from build123d import *

# Parameters (mm, degrees)
F1_DEPTH = 4
F2_R     = 3.5
F2_R_2   = 1.05
F3_DEPTH = 3


with BuildPart() as f1:
    # F0 (on Top) → F1 (new body)
    with BuildSketch(Plane.XY):
        with BuildLine():
            Line((2.511473671, -1.45), (2.511473671, 1.45))
            Line((2.511473671, 1.45), (0, 2.9))
            Line((0, 2.9), (0, 1.05))
            ThreePointArc((0, 1.05), (0.7424621202, 0.7424621202), (1.05, 0))
            ThreePointArc((1.05, 0), (0.7424621202, -0.7424621202), (0, -1.05))
            Line((0, -1.05), (0, -2.9))
            Line((0, -2.9), (2.511473671, -1.45))
        make_face()
        with BuildLine():
            Line((0, 1.05), (0, 2.9))
            Line((0, 2.9), (-2.511473671, 1.45))
            Line((-2.511473671, 1.45), (-2.511473671, -1.45))
            Line((-2.511473671, -1.45), (0, -2.9))
            Line((0, -2.9), (0, -1.05))
            ThreePointArc((0, -1.05), (-1.05, 0), (0, 1.05))
        make_face()
    extrude(amount=F1_DEPTH)

    # F2 (on face) → F3 (join)
    with BuildSketch(Plane(origin=(0, 0, 0), x_dir=(1, 0, 0), z_dir=(0, 0, -1))):
        Circle(F2_R)
        Polygon((0, 2.9), (2.511473671, 1.45), (2.511473671, -1.45), (0, -2.9), (-2.511473671, -1.45), (-2.511473671, 1.45), align=None, mode=Mode.SUBTRACT)
        Polygon((2.511473671, -1.45), (2.511473671, 1.45), (0, 2.9), (-2.511473671, 1.45), (-2.511473671, -1.45), (0, -2.9), align=None)
        Circle(F2_R_2, mode=Mode.SUBTRACT)
        Circle(F2_R_2)
    extrude(amount=F3_DEPTH)


solid = f1.part
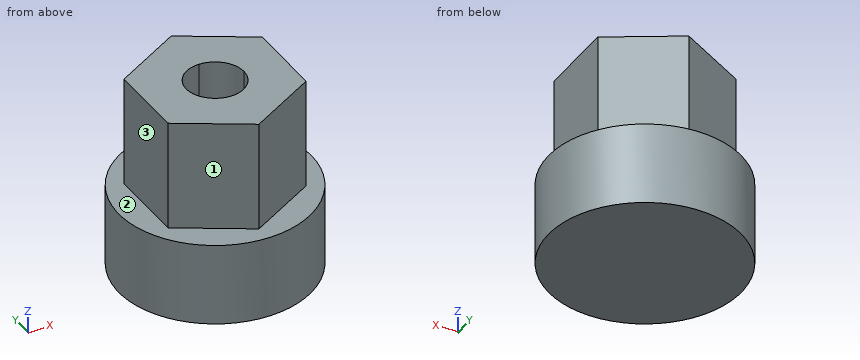
Could you check a few things on this model? Use its own coordinates, in mm. Face numbers are marked on the shaded views. A direction names the side the tool comes from. Give positions to 0.01 mm unless a question says otherwise; leave off trailing zeros. Order: outer loops, then holes, each group sorted by start corner. A loop starts at its lowest first (then second) coordinate and runs counter-clockwise, first axis right, second up.
Item 1: If we section it at C-C, the plane x = -0.5: Write out the boundary of the cut face in (y, z).
Item 2: If we section it at B-B, the plane y = 2.5: Write out the boundary of the cut face in (x, z).
Item 3: I need wall thicknesses on line 1 (X direction, y = 0, z = 2); line 2 (Z direction, x = -2, y = -2.5); line 3 (X direction, y = -1.25, z = 3.5). Which ranges of each line are inside material? Lowest first, please.
Item 4: For the marked faces 1, 2 and 3, which set-ups out of +Z, -Z, +X, -X, +Y, -Y let a thin tool reach every point of the face, with its end or its side?
Item 5: If we section it at A-A, the plane z = 2.75: Write out the boundary of the cut face in (x, y), plus the area to 3 significant figures.
Item 6: If we section it at D-D, the plane z = -2: Write out the boundary of the cut face in (x, y).
Item 7: I'm going to push flat-ended pins straight in: pin 1 (3 mm diameter, centred on x = 2, z = 1, fed in from -Y); pin 2 (1.5 mm diameter, centred on y = 1.5, z = 0, fed in from -X); pin 3 (1.4 mm diameter, centred on y = -0.5, z = 1, fed in from +X); pin 4 (2 mm diameter, centred on x = 2.5, y = -2.5, fed in from -Z). Where does each tip first touch, or does it pass through?
Values:
1. outline: (-3.46, -3) - (3.46, -3) - (3.46, 0) - (2.61, 0) - (2.61, 4) - (0.92, 4) - (0.92, 0) - (-0.92, 0) - (-0.92, 4) - (-2.61, 4) - (-2.61, 0) - (-3.46, 0) - close
2. outline: (-2.45, -3) - (2.45, -3) - (2.45, 0) - (0.69, 0) - (0.69, 4) - (-0.69, 4) - (-0.69, 0) - (-2.45, 0) - close
3. line 1: x = -2.51 to -1.05, 1.05 to 2.51
3. line 2: z = -3 to 0
3. line 3: x = -2.51 to 2.51
4. face 1: +Z, -X, -Y
4. face 2: +Z
4. face 3: +Z, -X, +Y, -Y
5. outline: (-2.51, -1.45) - (0, -2.9) - (2.51, -1.45) - (2.51, 1.45) - (0, 2.9) - (-2.51, 1.45) - close; hole circle Ø2.1 at (0, 0)
5. area: 18.4 mm2
6. outline: circle Ø7 at (0, 0)
7. pin 1: stops at y = -3.39
7. pin 2: stops at x = -3.42
7. pin 3: stops at x = 2.51
7. pin 4: stops at z = -3
